Here's how the part is built. I have some questions about the finished solid (model axes, mm). A direction names the side the tool comes from. Give positions to 0.01 mm unless a question says otherwise; leave off trailing zeros. Write each loop counter-clockwise with the first axis right and the second up, starting at its lowest first coordinate (ties: lowest second). Pieces come first, ordered by that corner, then holes. Notation, with made-up numbers: (39, 13.25) -> (54, 13.25) arc R25 cw to (54, 44.25) -> close; hole circle Ø10 at (-27.75, 85). An arc over 180 degrees is marked (long way). Use one line per item in the form item = value.
```python
from build123d import *

# Parameters (mm, degrees)
F2_DEPTH = 9.525


# Not quite as in the source:
# - a variable given as a bare number and used for a length is read in inches; the dataset says mm whatever the document's units were


with BuildPart() as f2:
    # F1 (on Top) → F2 (new body)
    with BuildSketch(Plane.XY):
        with BuildLine():
            Line((4.1244459855, 11.90625), (4.1244459855, 35.71875))
            ThreePointArc((4.1244459855, 35.71875), (0, 38.1), (-4.1244459855, 35.71875))
            Line((-4.1244459855, 35.71875), (-4.1244459855, 11.90625))
            Line((-4.1244459855, 11.90625), (0, 19.05))
            Line((0, 19.05), (4.1244459855, 11.90625))
        make_face()
        with BuildLine():
            Line((4.1244459855, 7.14375), (4.1244459855, 11.90625))
            Line((4.1244459855, 11.90625), (0, 19.05))
            Line((0, 19.05), (0, 7))
            Line((0, 7), (2, 7))
            Line((2, 7), (2, 4.582575695))
            ThreePointArc((2, 4.582575695), (4.1833001327, 2.7386127875), (5, 0))
            ThreePointArc((5, 0), (4.8296291314, -1.2940952255), (4.3301270189, -2.5))
            Line((4.3301270189, -2.5), (16.4977839421, -9.525))
            Line((16.4977839421, -9.525), (12.3733379566, -2.38125))
            Line((12.3733379566, -2.38125), (8.248891971, 0))
            Line((8.248891971, 0), (4.1244459855, 7.14375))
        make_face()
        with BuildLine():
            Line((0, 19.05), (-4.1244459855, 11.90625))
            Line((-4.1244459855, 11.90625), (-4.1244459855, 7.14375))
            Line((-4.1244459855, 7.14375), (-8.248891971, 0))
            Line((-8.248891971, 0), (-12.3733379566, -2.38125))
            Line((-12.3733379566, -2.38125), (-16.4977839421, -9.525))
            Line((-16.4977839421, -9.525), (-4.3301270189, -2.5))
            ThreePointArc((-4.3301270189, -2.5), (-4.7495627838, 1.562579074), (-2, 4.582575695))
            Line((-2, 4.582575695), (-2, 7))
            Line((-2, 7), (0, 7))
            Line((0, 7), (0, 19.05))
        make_face()
        with BuildLine():
            Line((4.1244459855, -7.14375), (8.248891971, -9.525))
            Line((8.248891971, -9.525), (16.4977839421, -9.525))
            Line((16.4977839421, -9.525), (4.3301270189, -2.5))
            ThreePointArc((4.3301270189, -2.5), (0, -5), (-4.3301270189, -2.5))
            Line((-4.3301270189, -2.5), (-16.4977839421, -9.525))
            Line((-16.4977839421, -9.525), (-8.248891971, -9.525))
            Line((-8.248891971, -9.525), (-4.1244459855, -7.14375))
            Line((-4.1244459855, -7.14375), (4.1244459855, -7.14375))
        make_face()
        with BuildLine():
            ThreePointArc((28.8711218987, -21.43125), (32.9955678842, -19.05), (32.9955678842, -14.2875))
            Line((32.9955678842, -14.2875), (12.3733379566, -2.38125))
            Line((12.3733379566, -2.38125), (16.4977839421, -9.525))
            Line((16.4977839421, -9.525), (8.248891971, -9.525))
            Line((8.248891971, -9.525), (28.8711218987, -21.43125))
        make_face()
        with BuildLine():
            Line((-12.3733379566, -2.38125), (-32.9955678842, -14.2875))
            ThreePointArc((-32.9955678842, -14.2875), (-32.9955678842, -19.05), (-28.8711218987, -21.43125))
            Line((-28.8711218987, -21.43125), (-8.248891971, -9.525))
            Line((-8.248891971, -9.525), (-16.4977839421, -9.525))
            Line((-16.4977839421, -9.525), (-12.3733379566, -2.38125))
        make_face()
        Polygon((-8.248891971, -9.525), (8.248891971, -9.525), (4.1244459855, -7.14375), (-4.1244459855, -7.14375), align=None)
        Polygon((12.3733379566, -2.38125), (4.1244459855, 11.90625), (4.1244459855, 7.14375), (8.248891971, 0), align=None)
        Polygon((-4.1244459855, 7.14375), (-4.1244459855, 11.90625), (-12.3733379566, -2.38125), (-8.248891971, 0), align=None)
    extrude(amount=F2_DEPTH)


solid = f2.part
```
Q1. I want a section at C-C, the plane y = -13. Write out the boundary of the cut face in (x, z) (3 decimals), and give its area (3 significant figures).
Result set:
outline = (-30.766, 0) -> (-14.268, 0) -> (-14.268, 9.525) -> (-30.766, 9.525) -> close; (14.268, 0) -> (30.766, 0) -> (30.766, 9.525) -> (14.268, 9.525) -> close
area = 314 mm2
Q2. I want a section at B-B, the plane x = -0.5. Write out the boundary of the cut face in (y, z) (3 decimals), and give its area (3 significant figures).
Result set:
outline = (-9.525, 0) -> (-4.975, 0) -> (-4.975, 9.525) -> (-9.525, 9.525) -> close; (7, 0) -> (38.074, 0) -> (38.074, 9.525) -> (7, 9.525) -> close
area = 339 mm2
Q3. Will these pins go through, and if not, where does the flat tip stop? pin 1 Ø5 at (x, z) = (1, 6) entering from -Y (3 decimals); pin 2 Ø1.5 at (y, z) = (21, 3) entering from -X; pin 3 Ø5 at (x, z) = (20.5, 6) entering from +Y.
Result set:
pin_1 = -9.525
pin_2 = -4.12
pin_3 = -5.63
Q4. I want a section at A-A, the plane z = 8.75. Write out the boundary of the cut face in (x, y) (1 decimal).
Result set:
outline = (-33, -14.3) arc R4.8 ccw to (-28.9, -21.4) -> (-8.2, -9.5) -> (8.2, -9.5) -> (28.9, -21.4) arc R4.8 ccw to (33, -14.3) -> (12.4, -2.4) -> (4.1, 11.9) -> (4.1, 35.7) arc R4.8 ccw to (-4.1, 35.7) -> (-4.1, 11.9) -> (-12.4, -2.4) -> close; hole (-2, 4.6) arc R5 ccw (long way) to (2, 4.6) -> (2, 7) -> (-2, 7) -> close
Q5. If I drill on line 1 along X through (y, z) = (34, 2.5); line 2 along X through (y, z) = (-16.5, 1); line 3 along X through (y, z) = (-10, 1), over which ranges is the centre line in solid material (lowest first)? Write a range as from..to.
Result set:
line_1 = -4.12..4.12
line_2 = -33.63..-20.33, 20.33..33.63
line_3 = -25.57..-9.07, 9.07..25.57
Q6. I want a section at D-D, the plane y = 33. Write out the boundary of the cut face in (x, z) (3 decimals).
Result set:
outline = (-4.124, 0) -> (4.124, 0) -> (4.124, 9.525) -> (-4.124, 9.525) -> close
Q7. If we mould it in two halves opening along Y, with no side actions, what happens to faces 1 (the face through (8.31, 4.66, 4.7)), 2 (the face through (-2, 6, 5)), 3 (the face through (2, 6, 5)), 4 (the face through (-33.03, -18.99, 4.7))? For each: +Y half, -Y half, draft (parallel to the pull), parting line (faces both ways), or undercut.
Result set:
face_1 = +Y half
face_2 = undercut
face_3 = undercut
face_4 = parting line
Q8. Which directions (+Z, -Z, +X, -X, +Y, -Y) give clear straight access to the entire face, cutting with the end or side of a thin tool? Please do faces 5 (the face through (18.416, -15.395, 4.696)), 6 (the face through (0, 7, 5)), 7 (the face through (4.124, 24, 5)).
Result set:
face_5 = +Z, -Z, -Y
face_6 = +Z, -Z
face_7 = +Z, -Z, +X, +Y
